Drawing for the job (mm, zero at the part's lowest x, y, z). A direction names the side the tool comes from. Coordinates: 2 decimals unless noted, no trailing zeros. Order: outer loops, then holes, each group sorted by start corner. A loop starts at its lowest first (then second) coordinate and runs counter-clockwise, first axis right, second up.
1) Pin check, flat tip, straight feed: pin 1 Ø1.5 at (x, y) = (2.5, 3) entering from +Z. Stop position of the tip, or through.
2) Mould opens along Y. For the marked faces 5, 6 and 7 say: +Y half, -Y half, draft (parallel to the pull), parting line (faces both ways), or undercut.
3) Cut at D-D (x = 3.8). List the corners of the cut face in (y, z).
4) Cut at C-C (z = 0.55). List the corners of the cut face in (x, y), and give its area (3 significant figures).
5) Wall check: L1, parallel to Y at x = 1.95, z = 4.8; L2, parallel to Y at x = 5.7, z = 2.15; L3, parallel to Y at x = 0.6, z = 2.9. Give the ranges that are in metal, low to high.
6) Cut at A-A (x = 0.5). List the corners of the cut face in (y, z).
7) Tool access for the marked faces 1, 2, 3 and 4: list every direction of +Z, -Z, +X, -X, +Y, -Y with a clear straight run to the whole face (end or side of a thin tool).
8) Cut at B-B (z = 4.2). List the corners of the cut face in (x, y).
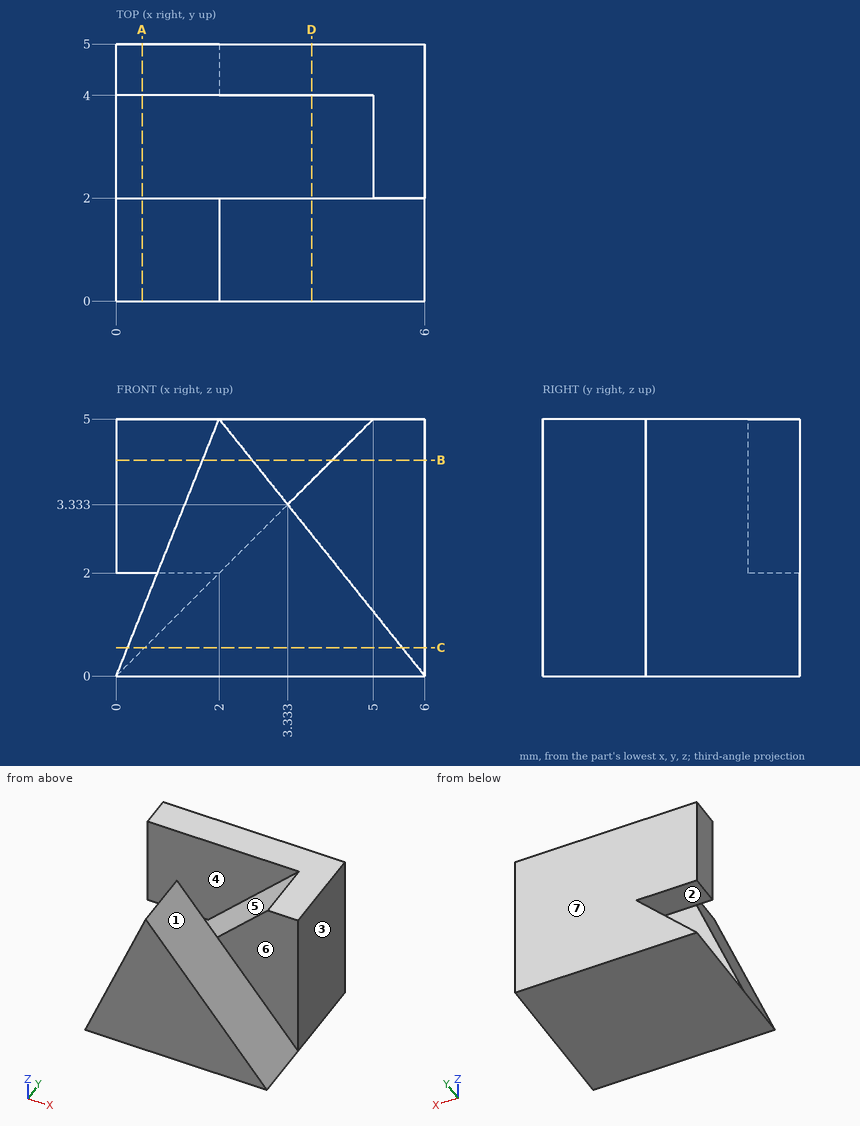
Geometry check:
1. pin 1: stops at z = 3.25
2. face 5: undercut
2. face 6: -Y half
2. face 7: +Y half
3. outline: (0, 0) - (5, 0) - (5, 5) - (4, 5) - (4, 3.8) - (2, 3.8) - (2, 2.75) - (0, 2.75) - close
4. outline: (0.22, 0) - (5.56, 0) - (5.56, 2) - (6, 2) - (6, 5) - (0.55, 5) - (0.55, 2) - (0.22, 2) - close
4. area: 27.0 mm2
5. L1: y = 0 to 2, 4 to 5
5. L2: y = 2 to 5
5. L3: y = 4 to 5
6. outline: (0, 0) - (5, 0) - (5, 0.5) - (2, 0.5) - (2, 1.25) - (0, 1.25) - close; (4, 2) - (5, 2) - (5, 5) - (4, 5) - close
7. face 1: +Z, +X, -Y
7. face 2: -X, +Y
7. face 3: +Z, -Z, +X, +Y, -Y
7. face 4: +Z, -X
8. outline: (0, 4) - (4.2, 4) - (4.2, 2) - (6, 2) - (6, 5) - (0, 5) - close; (1.68, 0) - (2.64, 0) - (2.64, 2) - (1.68, 2) - close
